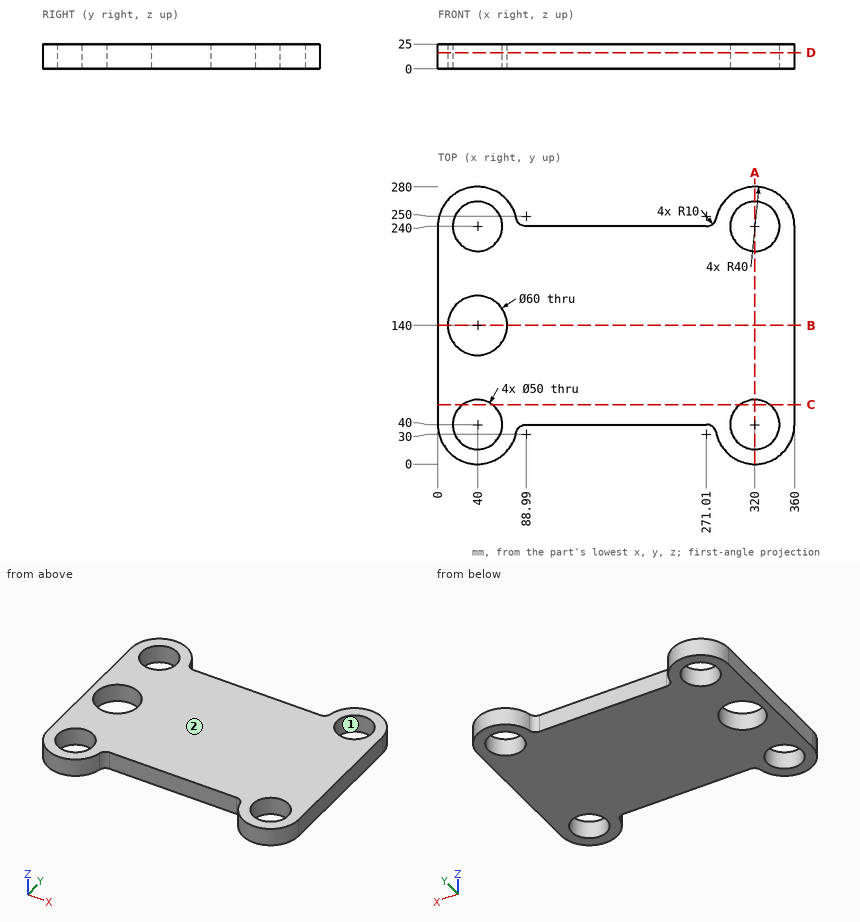
The drawing under review shows one solid part. Ordinate dimensions are in mm from its lowest x, y, z. Round coordinates to 2 decimals unless told otherwise and drop trailing zeros. Order: outer loops, then holes, each group sorted by start corner. A loop starts at its lowest first (then second) coordinate and runs counter-clockwise, first axis right, second up. Notation, with made-up numbers: (72.25, 67.5) -> (120.25, 67.5) arc R20 cw to (120.25, 103.5) -> close; hole circle Ø6 at (6, 0.25). An arc over 180 degrees is marked (long way). Use a Markdown table: item, result.
Item 1: Take a section at D-D (z = 16.25). State the section outline as (x, y) points, plus the area to 3 significant figures.
Resolved:
| item | result |
|---|---|
| outline | (0, 40) arc R40 ccw to (79.19, 32) arc R10 cw to (88.99, 40) -> (271.01, 40) arc R10 cw to (280.81, 32) arc R40 ccw to (360, 40) -> (360, 240) arc R40 ccw to (280.81, 248) arc R10 cw to (271.01, 240) -> (88.99, 240) arc R10 cw to (79.19, 248) arc R40 ccw to (0, 240) -> close; hole circle Ø60 at (40, 140); hole circle Ø50 at (40, 40); hole circle Ø50 at (40, 240); hole circle Ø50 at (320, 40); hole circle Ø50 at (320, 240) |
| area | 71,400 mm² |
Item 2: Take a section at C-C (y = 60). State the section outline as (x, z) points, plus the area to 3 significant figures.
Resolved:
| item | result |
|---|---|
| outline | (0, 0) -> (25, 0) -> (25, 25) -> (0, 25) -> close; (55, 0) -> (305, 0) -> (305, 25) -> (55, 25) -> close; (335, 0) -> (360, 0) -> (360, 25) -> (335, 25) -> close |
| area | 7,500 mm² |
Item 3: For line 1 along Y through (x, z) = (40, 12.75); line 2 along Y through (x, z) = (320, 7); line 3 along Y through (x, z) = (310, 19.75), list the stretches that pass through material, from the lowest coordinate up. Write a range as [from, to].
Resolved:
| item | result |
|---|---|
| line 1 | y = [0, 15], [65, 110], [170, 215], [265, 280] |
| line 2 | y = [0, 15], [65, 215], [265, 280] |
| line 3 | y = [1.27, 17.09], [62.91, 217.09], [262.91, 278.73] |
Item 4: For pin 1 (2 mm diameter, centred on x = 151, z = 5.5, fed in from +Y); pin 2 (6 mm diameter, centred on x = 304.5, z = 3.5, fed in from -Y), all flat-tipped, find the tip position at first contact; note any pin that passes through.
Resolved:
| item | result |
|---|---|
| pin 1 | stops at y = 240 |
| pin 2 | stops at y = 2 |
Item 5: Take a section at B-B (y = 140). State the section outline as (x, z) points, plus the area to 3 significant figures.
Resolved:
| item | result |
|---|---|
| outline | (0, 0) -> (10, 0) -> (10, 25) -> (0, 25) -> close; (70, 0) -> (360, 0) -> (360, 25) -> (70, 25) -> close |
| area | 7,500 mm² |
Item 6: Draft analysis for pull direction X (two halves, no side actions). For the marked faces 1 and 2, state which applies: +X half, -X half, draft (parallel to the pull), parting line (faces both ways), or undercut.
Resolved:
| item | result |
|---|---|
| face 1 | undercut |
| face 2 | draft |
Item 7: Take a section at A-A (x = 320). State the section outline as (y, z) points, plus the area to 3 significant figures.
Resolved:
| item | result |
|---|---|
| outline | (0, 0) -> (15, 0) -> (15, 25) -> (0, 25) -> close; (65, 0) -> (215, 0) -> (215, 25) -> (65, 25) -> close; (265, 0) -> (280, 0) -> (280, 25) -> (265, 25) -> close |
| area | 4,500 mm² |
